from build123d import *

# Parameters (mm, degrees)
SKETCH1_R                = 16.5
SKETCH1_R_2              = 8.15
BOSS_EXTRUDE1_DEPTH      = 8
SKETCH2_R                = 3
CUT_EXTRUDE1_DEPTH       = 25.667792767
TAP1_D                   = 2.459
CIRPATTERN11_OUTLINE_R   = 3
CIRPATTERN11_OUTLINE_R_2 = 1.2295
CIRPATTERN11_DEPTH       = 8
FILLET1_R                = 0.3


# Read off the part's stored shape, not the designer's step: CirPattern11
with BuildPart() as part:
    # Sketch1 → Boss-Extrude1 (new body)
    with BuildSketch(Plane.XY):
        Circle(SKETCH1_R)
        Circle(SKETCH1_R_2, mode=Mode.SUBTRACT)
    extrude(amount=BOSS_EXTRUDE1_DEPTH)

    # Sketch2 → Cut-Extrude1 (cut, through all)
    with BuildSketch(Plane.XY.offset(8)):
        with Locations((0, 12.5)):
            Circle(SKETCH2_R)
        with Locations((0, -12.5)):
            Circle(SKETCH2_R)
    extrude(amount=-CUT_EXTRUDE1_DEPTH, mode=Mode.SUBTRACT)

    # Tap1 (through all)
    with Locations(Plane.XY.offset(8)):
        with Locations((-12.5, 0), (12.5, 0)):
            Hole(TAP1_D / 2)

    # CirPattern11 outline → CirPattern11 (cut)
    with BuildSketch(Plane.XY):
        with Locations((8.838834765, 8.838834765)):
            Circle(CIRPATTERN11_OUTLINE_R)
        with Locations((-8.838834765, -8.838834765)):
            Circle(CIRPATTERN11_OUTLINE_R)
        with Locations((8.838834765, -8.838834765)):
            Circle(CIRPATTERN11_OUTLINE_R_2)
        with Locations((-8.838834765, 8.838834765)):
            Circle(CIRPATTERN11_OUTLINE_R_2)
    extrude(amount=CIRPATTERN11_DEPTH, mode=Mode.SUBTRACT)

    # Fillet1
    fillet1_edges = [part.edges().sort_by_distance(p)[0] for p in [
        (-16.5, 0, 0),
        (-16.5, 0, 8),
    ]]
    fillet(fillet1_edges, radius=FILLET1_R)


solid = part.part
Input: part model. Units: mm. Frame: model coordinates. Give positions to 0.01 mm unless a question says otherwise; leave off trailing zeros. Write each loop counter-clockwise with the first axis right and the second up, starting at its lowest first coordinate (ties: lowest second). Pieces come first, ordered by that corner, then holes.
Q1. Section A-A, the plane x = 0. Output: boundary loops of the cut face in (y, z), plus the area to 3 significant figures.
Q2. First-contact query: P1, Ø12, axis at x = 5, y = 1.5, coming from the +Z side; P2, Ø1.5, axis at x = -12.5, y = 0, coming from the -Z side; P3, Ø1, axis at x = 11, z = 4.5, coming from the +Y side; P4, Ø3, axis at y = 6, z = 5, coming from the +X side. Flat tips, straight axial feed; report the tip coordinate or a pass-through.
Q3. Section B-B, the plane z = 3.75. State how many separate pieces and enclosed holes the cut face has, plus the area to 3 significant figures.
Q4. Material intervals for probe 1 along Y at (x, z) = (-11.5, 2.25); probe 2 along X at (y, z) = (11, 2); probe 3 along Y at (x, z) = (7.5, 4), sorted ascending.
Q5. Pull-direction query (X, two-part tool) for faces 1 (the face through (-7.4, 3.8, 0)), 2 (the face through (-13.673, 0.369, 3.944)), 3 (the face through (15.24, -6.32, 3.95)); classes: pulls with the +X half, pulls with the -X half, needs draft (parallel to the pull), parting line crosses it, or undercut.
Filled in:
1. outline: (-16.5, 0.3) arc R0.3 ccw to (-16.2, 0) - (-15.5, 0) - (-15.5, 8) - (-16.2, 8) arc R0.3 ccw to (-16.5, 7.7) - close; (-9.5, 0) - (-8.15, 0) - (-8.15, 8) - (-9.5, 8) - close; (8.15, 0) - (9.5, 0) - (9.5, 8) - (8.15, 8) - close; (15.5, 0) - (16.2, 0) arc R0.3 ccw to (16.5, 0.3) - (16.5, 7.7) arc R0.3 ccw to (16.2, 8) - (15.5, 8) - close
1. area: 37.5 mm2
2. P1: stops at z = 8
2. P2: passes through
2. P3: stops at y = 12.73
2. P4: stops at x = 15.87
3. separate pieces: 1
3. enclosed holes: 9
3. area: 515 mm2
4. probe 1: y = -11.83 to -10.22, -7.45 to -0.72, 0.72 to 11.83
4. probe 2: x = -12.3 to -2.6, 2.6 to 6.76, 10.92 to 12.3
4. probe 3: y = -14.7 to -3.19, 3.19 to 6.15, 11.52 to 14.7
5. face 1: needs draft
5. face 2: undercut
5. face 3: parting line crosses it
